from build123d import *

# Parameters (mm, degrees)
F0_W     = 78.535166
F0_H     = 128.679674
F1_DEPTH = 25.4
F2_R     = 5.08
F3_R     = 5.08
F4_R     = 5.08
F5_R     = 5.08
F6_T     = -2819.4
F8_DEPTH = 25.4


with BuildPart() as f1:
    # F0 (on Front) → F1 (new body)
    with BuildSketch(Plane.XZ):
        with Locations((-4.977578, 3.318386)):
            Rectangle(F0_W, F0_H)
    extrude(amount=F1_DEPTH)

    # F2
    f2_edges = [f1.edges().sort_by_distance(p)[0] for p in [
        (-4.977578, -25.4, 67.658223),
    ]]
    fillet(f2_edges, radius=F2_R)

    # F3
    f3_edges = [f1.edges().sort_by_distance(p)[0] for p in [
        (-44.245161, -25.4, 0.778386),
    ]]
    fillet(f3_edges, radius=F3_R)

    # F4
    f4_edges = [f1.edges().sort_by_distance(p)[0] for p in [
        (34.290005, -25.4, 0.778386),
    ]]
    fillet(f4_edges, radius=F4_R)

    # F5
    f5_edges = [f1.edges().sort_by_distance(p)[0] for p in [
        (-4.977578, -25.4, -61.021451),
    ]]
    fillet(f5_edges, radius=F5_R)

    # F6
    f6_openings = [f1.faces().sort_by_distance(p)[0] for p in [
        (-4.977578, -25.4, 3.318386),
    ]]
    offset(amount=F6_T, openings=f6_openings)

    # F7 (on Front) → F8 (cut)
    with BuildSketch(Plane.XZ):
        Polygon((5.745283, -2.317451), (6.463282, 18.76704), (-21.526827, 16.971201), (-24.241816, 0), align=None)
    extrude(amount=F8_DEPTH, mode=Mode.SUBTRACT)


solid = f1.part
Can you work these out from the model? Positions are in its coordinate system, mm. A direction names the side the tool comes from. Round coordinates to 2 decimals unless told otherwise and drop trailing zeros. Write each loop counter-clockwise with the first axis right and the second up, starting at its lowest first coordinate (ties: lowest second). Pieces come first, ordered by that corner, then holes. Notation, with made-up numbers: (-1, 31.25) -> (50, 31.25) arc R19 ccw to (50, 51.25) -> close; hole circle Ø8 at (34, -8). An arc over 180 degrees is marked (long way). Use one line per item in the form item = value. Start each with the question number.
Q1. We'd pull the mould along Z, two halves only. Please class faces 3 (the face through (-22.865, -12.522, 8.604)), 4 (the face through (32.84, -10.02, 66.13)), 5 (the face through (-42.8, -23.87, 4.15)): +Z half, -Z half, draft (parallel to the pull), parting line (faces both ways), or undercut.
Q2. Which directions (+Z, -Z, +X, -X, +Y, -Y) give clear straight access to the entire face, cutting with the end or side of a thin tool? Please do faces 1 (the face through (-9.458, -12.522, -1.143)), 2 (the face through (-42.797, -10.018, 66.131)).
Q3. Imagine slicing it at B-B (x = -10). Please give me the cut outline in (y, z), then the cut area to 3 significant figures.
Q4. If I drill on probe 1 along Z at (x, y) = (-8, -8.25); probe 2 along Z at (x, y) = (-39.5, -15.25); probe 3 along Z at (x, y) = (1.5, -21), over which ranges is the centre line in solid material (lowest first)? Write a range as [from, to].
Q5. Imagine slicing it at A-A (y = -5). Please give me the cut outline in (x, z).
Q6. Imagine slicing it at C-C (z = 13). Please give me the cut outline in (x, y).
Worked out:
q1.face_3 = undercut
q1.face_4 = +Z half
q1.face_5 = draft
q2.face_1 = +Y, -Y
q2.face_2 = +Z, -X, +Y, -Y
q3.outline = (-25.4, -55.94) arc R5.08 ccw to (-20.32, -61.02) -> (0, -61.02) -> (0, -1.1) -> (-25.4, -1.1) -> close; (-25.4, 17.71) -> (0, 17.71) -> (0, 67.66) -> (-20.32, 67.66) arc R5.08 ccw to (-25.4, 62.58) -> close
q3.area = 2,780 mm^2
q4.probe_1 = [-61.02, -1.26], [17.84, 67.66]
q4.probe_2 = [-61.01, 67.65]
q4.probe_3 = [-60.98, -1.99], [18.45, 67.61]
q5.outline = (-44.25, -55.94) arc R5.08 ccw to (-39.17, -61.02) -> (29.21, -61.02) arc R5.08 ccw to (34.29, -55.94) -> (34.29, 62.58) arc R5.08 ccw to (29.21, 67.66) -> (-39.17, 67.66) arc R5.08 ccw to (-44.25, 62.58) -> close; hole (-24.24, 0) -> (5.75, -2.32) -> (6.46, 18.77) -> (-21.53, 16.97) -> close
q6.outline = (-44.25, -20.32) arc R5.08 ccw to (-39.17, -25.4) -> (-22.16, -25.4) -> (-22.16, 0) -> (-44.25, 0) -> close; (6.27, -25.4) -> (29.21, -25.4) arc R5.08 ccw to (34.29, -20.32) -> (34.29, 0) -> (6.27, 0) -> close
